The listing builds one solid part. Answer for the finished solid, in the listing's coordinates (mm). A direction names the side the tool comes from. Give positions to 0.01 mm unless a question says otherwise; leave off trailing zeros. Write each loop counter-clockwise with the first axis right and the second up, starting at its lowest first coordinate (ties: lowest second). Pieces come first, ordered by that corner, then holes. Notation, with made-up numbers: M -1,-8.5 L 35,-8.5 A13 ccw 35,-0.5 Z; hole C -40,73 d2. An arc over 180 degrees is marked long. Answer as a JSON object with one key per item and string values.
```python
from build123d import *

# Parameters (mm, degrees)
SKETCH1_W                   = 51
SKETCH1_H                   = 38
SKETCH1_W_2                 = 41
SKETCH1_H_2                 = 21
MAIN_BODY_DEPTH             = 10
SKETCH2_W                   = 41
SKETCH2_H                   = 21
SKETCH2_W_2                 = 39
SKETCH2_H_2                 = 19
MID_SERVO_GAP_DEPTH         = 5
EDGE_CONTOURING_R           = 1
SKETCH3_W                   = 13
SKETCH3_H                   = 7
AIRWAY_DEPTH                = 52
SKETCH4_W                   = 15
SKETCH4_H                   = 5.5
CLEARANCE_CABLES_DEPTH      = 21
CONTOURING_OUTER_R          = 3
CONTOURING_AIRWAY_R         = 1
CONTOURING_INNER_R          = 2.5
CLEARANCE_SERVO_INSERTION_R = 1


with BuildPart() as part:
    # Sketch1 → Main Body (new body, symmetric)
    with BuildSketch(Plane(origin=(0, 0, 0), x_dir=(0, 0, -1), z_dir=(1, 0, 0))):
        Rectangle(SKETCH1_W, SKETCH1_H)
        Rectangle(SKETCH1_W_2, SKETCH1_H_2, mode=Mode.SUBTRACT)
    extrude(amount=MAIN_BODY_DEPTH, both=True)

    # Sketch2 → Mid Servo Gap (add, symmetric)
    with BuildSketch(Plane(origin=(0, 0, 0), x_dir=(0, 0, -1), z_dir=(1, 0, 0))):
        Rectangle(SKETCH2_W, SKETCH2_H)
        Rectangle(SKETCH2_W_2, SKETCH2_H_2, mode=Mode.SUBTRACT)
    extrude(amount=MID_SERVO_GAP_DEPTH, both=True)

    # Edge Contouring
    edge_contouring_edges = [part.edges().sort_by_distance(p)[0] for p in [
        (7.5, 10.5, 20.5),
        (7.5, -10.5, 20.5),
        (7.5, -10.5, -20.5),
        (7.5, 10.5, -20.5),
        (-7.5, 10.5, -20.5),
        (-7.5, 10.5, 20.5),
        (-7.5, -10.5, -20.5),
        (-7.5, -10.5, 20.5),
        (0, 9.5, 19.5),
        (0, -9.5, 19.5),
        (0, 9.5, -19.5),
    ]]
    fillet(edge_contouring_edges, radius=EDGE_CONTOURING_R)

    # Sketch3 → Airway (cut, through all)
    with BuildSketch(Plane.XY.offset(25.5)):
        Rectangle(SKETCH3_W, SKETCH3_H)
    extrude(amount=-AIRWAY_DEPTH, mode=Mode.SUBTRACT)

    # Sketch4 → Clearance - Cables (cut, through all)
    with BuildSketch(Plane(origin=(10, 0, 0), x_dir=(0, 0, -1), z_dir=(1, 0, 0))):
        with Locations((0, 16.25)):
            Rectangle(SKETCH4_W, SKETCH4_H)
        with Locations((0, -16.25)):
            Rectangle(SKETCH4_W, SKETCH4_H)
    extrude(amount=-CLEARANCE_CABLES_DEPTH, mode=Mode.SUBTRACT)

    # Contouring - Outer
    contouring_outer_edges = [part.edges().sort_by_distance(p)[0] for p in [
        (0, 19, 25.5),
        (0, 19, -25.5),
        (0, -19, -25.5),
        (0, -19, 25.5),
    ]]
    fillet(contouring_outer_edges, radius=CONTOURING_OUTER_R)

    # Contouring - Airway
    contouring_airway_edges = [part.edges().sort_by_distance(p)[0] for p in [
        (-6.5, -3.5, 23),
        (6.5, 3.5, 23),
        (-6.5, 3.5, 23),
        (6.5, -3.5, 23),
        (-6.5, -3.5, -23),
        (-6.5, 3.5, -23),
        (6.5, 3.5, -23),
        (6.5, -3.5, -23),
    ]]
    fillet(contouring_airway_edges, radius=CONTOURING_AIRWAY_R)

    # Contouring - Inner
    contouring_inner_edges = [part.edges().sort_by_distance(p)[0] for p in [
        (0, 13.5, 7.5),
        (0, 19, 7.5),
        (0, 19, -7.5),
        (0, 13.5, -7.5),
        (0, -19, -7.5),
        (0, -19, 7.5),
        (0, -13.5, 7.5),
        (0, -13.5, -7.5),
    ]]
    fillet(contouring_inner_edges, radius=CONTOURING_INNER_R)

    # Clearance - Servo Insertion
    clearance_servo_insertion_edges = [part.edges().sort_by_distance(p)[0] for p in [
        (-10, -10.5, 0),
        (-10, 0, -20.5),
        (-10, 0, 20.5),
        (10, 0, -20.5),
        (10, 10.5, 0),
        (-10, 10.5, 0),
        (10, 0, 20.5),
        (10, -10.5, 0),
        (-10, -10.207106781, -20.207106781),
        (-10, -10.207106781, 20.207106781),
        (10, 10.207106781, -20.207106781),
        (-10, 10.207106781, -20.207106781),
        (-10, 10.207106781, 20.207106781),
        (10, 10.207106781, 20.207106781),
        (10, -10.207106781, 20.207106781),
        (10, -10.207106781, -20.207106781),
    ]]
    fillet(clearance_servo_insertion_edges, radius=CLEARANCE_SERVO_INSERTION_R)


solid = part.part
```
1. For faces 1 (the flat face through (7, 10.5, 0)), 2 (the flat face through (0, -3.5, 23)), 3 (the cylindrical face through (0, 18, 8)), 4 (the cylindrical face through (0, -18, -8)), determine the directions among +Z, -Z, +X, -X, +Y, -Y from which every point of the face is accessible in a straight line to the end or side of a thin tool.
Verdict:
{"face 1": "+X", "face 2": "+Z, -Z", "face 3": "+X, -X, +Y", "face 4": "+X, -X, -Y"}
2. A cutting plane is placed at A-A, the plane y = -5. Give the vertices of the cut face in (x, z), plus the area to 3 significant figures.
Verdict:
{"outline": "M -10,-25.5 L 10,-25.5 L 10,-21.5 A1 ccw 9,-20.5 L 5,-20.5 L 5,-19.5 L -5,-19.5 L -5,-20.5 L -9,-20.5 A1 ccw -10,-21.5 Z; M -10,21.5 A1 ccw -9,20.5 L -5,20.5 L -5,19.5 L 5,19.5 L 5,20.5 L 9,20.5 A1 ccw 10,21.5 L 10,25.5 L -10,25.5 Z", "area": "219 mm2"}
3. Flat-ended cylindrical pins translate along their axes: pin 1 (3 mm diameter, centred on x = 1.5, z = 2, fed in from +Y); pin 2 (5 mm diameter, centred on y = -11, z = 1.5, fed in from -X); pin 3 (3 mm diameter, centred on x = -7, z = 4.5, fed in from -Y); pin 4 (3 mm diameter, centred on x = 4.5, z = 0.5, fed in from -Y). Find the tip coordinate at first contact, or state that the pin passes through.
Verdict:
{"pin 1": "stops at y = 13.5", "pin 2": "stops at x = -10", "pin 3": "stops at y = -13.71", "pin 4": "stops at y = -13.5"}
4. The mould has two halves that part along Z. Classify faces 5 (the cylindrical face through (-0.14, 18.14, -24.6)), 6 (the cylindrical face through (-0.14, 18.1, 24.64)), 7 (the flat face through (-10, 13, 0)), 8 (the cylindrical face through (-0.14, 14.252, 6.787)): released by +Z, released by -Z, zero draft, split by the parting line, or undercut.
Verdict:
{"face 5": "released by -Z", "face 6": "released by +Z", "face 7": "zero draft", "face 8": "undercut"}
5. A cutting plane is placed at B-B, the plane z = 11. Give the vertices of the cut face in (x, y).
Verdict:
{"outline": "M -10,-19 L 10,-19 L 10,-11.5 A1 ccw 9,-10.5 L 5,-10.5 L 5,-9.5 L -5,-9.5 L -5,-10.5 L -9,-10.5 A1 ccw -10,-11.5 Z; M -10,11.5 A1 ccw -9,10.5 L -5,10.5 L -5,9.5 L 5,9.5 L 5,10.5 L 9,10.5 A1 ccw 10,11.5 L 10,19 L -10,19 Z"}
6. A cutting plane is placed at D-D, the plane y = 0. Give the vertices of the cut face in (x, z).
Verdict:
{"outline": "M -10,-25.5 L -6.5,-25.5 L -6.5,-20.5 L -9,-20.5 A1 ccw -10,-21.5 Z; M -10,21.5 A1 ccw -9,20.5 L -6.5,20.5 L -6.5,25.5 L -10,25.5 Z; M 6.5,-25.5 L 10,-25.5 L 10,-21.5 A1 ccw 9,-20.5 L 6.5,-20.5 Z; M 6.5,20.5 L 9,20.5 A1 ccw 10,21.5 L 10,25.5 L 6.5,25.5 Z"}
7. Consider line 1 along Y through (x, z) = (3.5, 1); line 2 along Y through (x, z) = (9, 12); line 3 along Z through (x, y) = (-1.5, 8.5). Determine where each line is inside the solid, lowest interval first.
Verdict:
{"line 1": "y = -13.5 to -9.5, 9.5 to 13.5", "line 2": "y = -19 to -10.5, 10.5 to 19", "line 3": "z = -25.5 to -19.5, 19.5 to 25.5"}
